Geometry check sheet. Reference: the model listing, model coordinates, mm. A direction names the side the tool comes from. Coordinates: 2 decimals unless noted, no trailing zeros. Order: outer loops, then holes, each group sorted by start corner. A loop starts at its lowest first (then second) coordinate and runs counter-clockwise, first axis right, second up. Notation, with made-up numbers: (76.5, 67) -> (134.5, 67) arc R19 cw to (134.5, 101) -> close; hole circle Ø5 at (52.5, -39). An arc over 180 degrees is marked (long way). Answer in a Markdown table with one row per item. Add a question column.
```python
from build123d import *

# Parameters (mm, degrees)
BOSS_EXTRUDE1_DEPTH = 25
CUT_EXTRUDE1_DEPTH  = 88.424252928
CUT_EXTRUDE2_DEPTH  = 9
FILLET3_R           = 4


with BuildPart() as part:
    # Sketch1 → Boss-Extrude1 (new body)
    with BuildSketch(Plane(origin=(0, 0, 0), x_dir=(1, 0, 0), z_dir=(0, 1, 0))):
        Polygon((0, 0), (0, 33), (59, 33), (59, 9), (77, 9), (77, 0), align=None)
    extrude(amount=BOSS_EXTRUDE1_DEPTH)

    # Sketch3 → Cut-Extrude1 (cut, through all)
    with BuildSketch(Plane(origin=(0, 0, -33), x_dir=(-1, 0, 0), z_dir=(0, 0, -1))):
        with BuildLine():
            Line((-57, 0), (-2, 0))
            Line((-2, 0), (-2, 21))
            ThreePointArc((-2, 21), (-2.585786438, 22.414213562), (-4, 23))
            Line((-4, 23), (-55, 23))
            ThreePointArc((-55, 23), (-56.414213562, 22.414213562), (-57, 21))
            Line((-57, 21), (-57, 0))
        make_face()
    extrude(amount=-CUT_EXTRUDE1_DEPTH, mode=Mode.SUBTRACT)

    # Sketch4 → Cut-Extrude2 (cut)
    with BuildSketch(Plane.XY):
        with BuildLine():
            Line((75, 0), (51.080310893, 0))
            Line((51.080310893, 0), (51.080310893, 23))
            Line((51.080310893, 23), (73, 23))
            ThreePointArc((73, 23), (74.414213562, 22.414213562), (75, 21))
            Line((75, 21), (75, 0))
        make_face()
    extrude(amount=-CUT_EXTRUDE2_DEPTH, mode=Mode.SUBTRACT)

    # Fillet3
    # the kernel refuses this fillet: 4 mm, written as the material it takes off along each edge
    with BuildSketch(Plane(origin=(59, 25, -43), x_dir=(-1, 0, 0), z_dir=(0, 0, 1))) as fillet3_piece_1:
        with BuildLine():
            CenterArc((FILLET3_R, FILLET3_R), FILLET3_R, 180, 90)
            Line((0, FILLET3_R), (0, 0))
            Line((0, 0), (FILLET3_R, 0))
        make_face()
    extrude(amount=34, mode=Mode.SUBTRACT)
    with BuildSketch(Plane(origin=(0, 25, 10), x_dir=(0, -1, 0), z_dir=(0, 0, -1))) as fillet3_piece_2:
        with BuildLine():
            CenterArc((FILLET3_R, -FILLET3_R), FILLET3_R, 90, 90)
            Line((0, -FILLET3_R), (0, 0))
            Line((0, 0), (FILLET3_R, 0))
        make_face()
    extrude(amount=53, mode=Mode.SUBTRACT)
    with BuildSketch(Plane(origin=(77, 25, -19), x_dir=(-1, 0, 0), z_dir=(0, 0, 1))) as fillet3_piece_3:
        with BuildLine():
            CenterArc((FILLET3_R, FILLET3_R), FILLET3_R, 180, 90)
            Line((0, FILLET3_R), (0, 0))
            Line((0, 0), (FILLET3_R, 0))
        make_face()
    extrude(amount=29, mode=Mode.SUBTRACT)


solid = part.part
```
(1) Mould release check, pull along X, two halves, no side actions. Record for faces 4 (the face through (31, 25, -17)), 5 (the face through (30, 23, -16)), 6 (the face through (75.859, 23.797, -4.563)), 7 (the face through (2, 10, -17)): +X half, -X half, draft (parallel to the pull), parting line (faces both ways), or undercut.
(2) Access from +Z, -Z, +X, -X, +Y, -Y to the whole of each face (thin tool, end or side, straight path). Record for faces 1 (the face through (57.859, 23.797, -21.168)), 2 (the face through (58, 12, -9)), 3 (the face through (75, 11, -4)).
(3) Cross-section at C-C (x = 45). Enter the section's corners in (y, z).
(4) Cross-section at A-A (y = 9.5). Enter the section's corners in (x, z).
(5) Go/stop test with flat-tipped pins: P1, Ø1.5, axis at y = 5.5, z = -12.5, coming from the +X side; P2, Ø10, axis at x = 11, y = 14.5, coming from the -Z side; P3, Ø5, axis at x = 61, y = 5.5, coming from the +Z side. Record where each tip stops, or that it passes through.
(6) Scan lines: line 1 along X through (y, z) = (9.5, -1.5); line 2 along X through (y, z) = (10, -23.5); line 3 along Y through (x, z) = (45, -20). Record each from-to range of solid material in increasing order.
(7) Cross-section at B-B (z = -1.5). Enter the section's corners in (x, y), plus the area to 3 significant figures.
(8) Cross-section at D-D (z = -25.5). Enter the section's corners in (x, y).
Checks:
| question | item | result |
|---|---|---|
| 1 | face 4 | draft |
| 1 | face 5 | undercut |
| 1 | face 6 | +X half |
| 1 | face 7 | undercut |
| 2 | face 1 | -Z, +X, +Y |
| 2 | face 2 | +Z, -Y |
| 2 | face 3 | +Z, -Z, -Y |
| 3 | outline | (23, -33) -> (25, -33) -> (25, 0) -> (23, 0) -> close |
| 4 | outline | (0, -33) -> (2, -33) -> (2, 0) -> (0, 0) -> close; (57, -33) -> (59, -33) -> (59, -9) -> (57, -9) -> close; (75, -9) -> (77, -9) -> (77, 0) -> (75, 0) -> close |
| 5 | P1 | x = 59 |
| 5 | P2 | through |
| 5 | P3 | z = -9 |
| 6 | line 1 | 0 to 2, 75 to 77 |
| 6 | line 2 | 0 to 2, 57 to 59 |
| 6 | line 3 | 23 to 25 |
| 7 | outline | (0, 0) -> (2, 0) -> (2, 21) arc R2 cw to (4, 23) -> (73, 23) arc R2 cw to (75, 21) -> (75, 0) -> (77, 0) -> (77, 21) arc R4 ccw to (73, 25) -> (4, 25) arc R4 ccw to (0, 21) -> close |
| 7 | area | 241 mm² |
| 8 | outline | (0, 0) -> (2, 0) -> (2, 21) arc R2 cw to (4, 23) -> (55, 23) arc R2 cw to (57, 21) -> (57, 0) -> (59, 0) -> (59, 21) arc R4 ccw to (55, 25) -> (4, 25) arc R4 ccw to (0, 21) -> close |
